```python
from build123d import *

# Parameters (mm, degrees)
F0_W      = 43
F0_H      = 32
F0_W_2    = 39
F0_H_2    = 28
F1_DEPTH  = 16
F2_W      = 43
F2_H      = 32
F3_DEPTH  = 1.5
F4_W      = 10
F4_H      = 13.5
F5_DEPTH  = 2
F6_R      = 2
F7_DEPTH  = 1.5
F8_W      = 12
F8_H      = 16
F9_DEPTH  = 2
F10_W     = 15
F10_H     = 12
F11_DEPTH = 2
F12_W     = 10
F12_H     = 4
F13_DEPTH = 4
F14_W     = 10
F14_H     = 4
F15_DEPTH = 4


with BuildPart() as f1:
    # F0 (on Top) → F1 (new body)
    with BuildSketch(Plane.XY):
        with Locations((19.5, -14)):
            Rectangle(F0_W, F0_H)
        with Locations((19.5, -14)):
            Rectangle(F0_W_2, F0_H_2, mode=Mode.SUBTRACT)
    extrude(amount=F1_DEPTH)

    # F2 (on face) → F3 (join)
    with BuildSketch(Plane.XY.offset(16)):
        with Locations((19.5, -14)):
            Rectangle(F2_W, F2_H)
    extrude(amount=F3_DEPTH)

    # F4 (on face) → F5 (cut, through all)
    with BuildSketch(Plane(origin=(-2, 0, 0), x_dir=(0, -1, 0), z_dir=(-1, 0, 0))):
        with Locations((7, 6.75)):
            Rectangle(F4_W, F4_H)
    extrude(amount=-F5_DEPTH, mode=Mode.SUBTRACT)

    # F6 (on face) → F7 (cut, through all)
    with BuildSketch(Plane.XY.offset(17.5)):
        with Locations((2, -2)):
            Circle(F6_R)
    extrude(amount=-F7_DEPTH, mode=Mode.SUBTRACT)

    # F8 (on face) → F9 (cut, through all)
    with BuildSketch(Plane(origin=(0, 2, 0), x_dir=(-1, 0, 0), z_dir=(0, 1, 0))):
        with Locations((-32, 8)):
            Rectangle(F8_W, F8_H)
    extrude(amount=-F9_DEPTH, mode=Mode.SUBTRACT)

    # F10 (on face) → F11 (cut, through all)
    with BuildSketch(Plane.XZ.offset(30)):
        with Locations((28.5, 6)):
            Rectangle(F10_W, F10_H)
    extrude(amount=-F11_DEPTH, mode=Mode.SUBTRACT)

    # F12 (on face) → F13 (join)
    with BuildSketch(Plane.XZ.offset(30)):
        with Locations((16, 2)):
            Rectangle(F12_W, F12_H)
    extrude(amount=F13_DEPTH)

    # F14 (on face) → F15 (join)
    with BuildSketch(Plane(origin=(0, 2, 0), x_dir=(-1, 0, 0), z_dir=(0, 1, 0))):
        with Locations((-16, 2)):
            Rectangle(F14_W, F14_H)
    extrude(amount=F15_DEPTH)


solid = f1.part
```
Verification items for the finished model (mm, model axes). A direction names the side the tool comes from. Round coordinates to 2 decimals unless told otherwise and drop trailing zeros. Write each loop counter-clockwise with the first axis right and the second up, starting at its lowest first coordinate (ties: lowest second). Pieces come first, ordered by that corner, then holes. Notation, with made-up numbers: (31, 89.5) - (88, 89.5) arc R18 ccw to (88, 116.5) - close; hole circle Ø7 at (44, -5.5). An arc over 180 degrees is marked (long way). Answer as a JSON object with one key per item and string values. Group by question number.
Q1. Go/stop test with flat-tipped pins: pin 1 Ø2 at (x, y) = (13.5, 4.5) entering from +Z; pin 2 Ø2 at (y, z) = (-33, 2) entering from -X; pin 3 Ø1 at (x, y) = (30, -29.5) entering from -Z. Record where each tip stops, or that it passes through.
Q2. Thickness scan on line 1 (Y direction, x = 2, z = 17.1); line 2 (X direction, y = -2, z = 17.1); line 3 (Y direction, x = 11, z = 9.75). Record the ranges inside material, lowest first.
Q3. Tool access check on faces 1 (the flat face through (11, -32, 2)), 2 (the flat face through (36, -29, 6)), 3 (the flat face through (15, -28, 8)), 4 (the flat face through (21, 4, 2)), 5 (the flat face through (38, 1, 8)). Record the directions out of +Z, -Z, +X, -X, +Y, -Y that give a thin tool (end or side, any length) a straight path to the whole face; none if there is none.
Q4. Mould release check, pull along Y, two halves, no side actions. Record for faces 6 (the flat face through (-1, -12, 7)), 7 (the flat face through (16, -34, 2)), 8 (the flat face through (16, 4, 4)): released by +Y, released by -Y, zero draft, split by the parting line, or undercut.
Q5. Section check A-A, the plane z = 13. Enter the section's corners in (x, y), plus the area to 3 significant figures.
Q6. Section check B-B, the plane y = -21.5. Enter the section's corners in (x, z), plus the area to 4 significant figures.
Q7. Section check D-D, the plane z = 5.25. Enter the section's corners in (x, y).
Q8. Section check C-C, the plane x = 2.5. Enter the section's corners in (y, z).
Found:
{
 "1": {"pin 1": "stops at z = 4", "pin 2": "stops at x = 11", "pin 3": "stops at z = 12"},
 "2": {"line 1": "y = -30 to -4, 0 to 2", "line 2": "x = -2 to 0, 4 to 41", "line 3": "y = -30 to -28, 0 to 2"},
 "3": {"face 1": "+Z, -Z, -X, -Y", "face 2": "-Z, +Y, -Y", "face 3": "-Z", "face 4": "+Z, -Z, +X, +Y", "face 5": "-Z, +Y"},
 "4": {"face 6": "undercut", "face 7": "released by -Y", "face 8": "zero draft"},
 "5": {"outline": "(-2, -30) - (41, -30) - (41, 2) - (38, 2) - (38, 0) - (39, 0) - (39, -28) - (0, -28) - (0, -12) - (-2, -12) - close; (-2, -2) - (0, -2) - (0, 0) - (26, 0) - (26, 2) - (-2, 2) - close", "area": "240 mm^2"},
 "6": {"outline": "(-2, 0) - (0, 0) - (0, 16) - (39, 16) - (39, 0) - (41, 0) - (41, 17.5) - (-2, 17.5) - close", "area": "128.5 mm^2"},
 "7": {"outline": "(-2, -30) - (21, -30) - (21, -28) - (0, -28) - (0, -12) - (-2, -12) - close; (-2, -2) - (0, -2) - (0, 0) - (26, 0) - (26, 2) - (-2, 2) - close; (36, -30) - (41, -30) - (41, 2) - (38, 2) - (38, 0) - (39, 0) - (39, -28) - (36, -28) - close"},
 "8": {"outline": "(-30, 0) - (-28, 0) - (-28, 16) - (-3.94, 16) - (-3.94, 17.5) - (-30, 17.5) - close; (-0.06, 16) - (0, 16) - (0, 0) - (2, 0) - (2, 17.5) - (-0.06, 17.5) - close"}
}
